```python
from build123d import *

# Parameters (mm, degrees)
BOSS_EXTRUDE1_DEPTH            = 43
BOSS_EXTRUDE2_DEPTH            = 33
SKETCH6_R                      = 11
CUT_EXTRUDE1_DEPTH             = 2
SKETCH7_R                      = 2.5
CUT_EXTRUDE2_DEPTH             = 4
CBORE_FOR_M3_SHCS1_D           = 3.4
CBORE_FOR_M3_SHCS1_CBORE_D     = 6.5
CBORE_FOR_M3_SHCS1_CBORE_DEPTH = 3
CBORE_FOR_M3_SHCS2_D           = 3.4
CBORE_FOR_M3_SHCS2_CBORE_D     = 6.5
CBORE_FOR_M3_SHCS2_CBORE_DEPTH = 3
CBORE_FOR_M3_SHCS3_D           = 3.4
CBORE_FOR_M3_SHCS3_CBORE_D     = 6.5
CBORE_FOR_M3_SHCS3_CBORE_DEPTH = 3


with BuildPart() as part:
    # Sketch1 → Boss-Extrude1 (new body)
    with BuildSketch(Plane.XY):
        Polygon((-51.369142857, 0), (-21.369142857, 0), (-21.369142857, 33), (21.630857143, 33), (21.630857143, 0), (51.630857143, 0), (51.630857143, 9), (25.630857143, 9), (25.630857143, 38), (-25.369142857, 38), (-25.369142857, 9), (-51.369142857, 9), align=None)
    extrude(amount=BOSS_EXTRUDE1_DEPTH)

    # Sketch5 → Boss-Extrude2 (add)
    with BuildSketch(Plane.XZ.offset(-33)):
        Polygon((-21.369142857, 43), (-18.369142857, 43), (-21.369142857, 40), align=None)
        Polygon((21.630857143, 40), (21.630857143, 43), (18.630857143, 43), align=None)
        Polygon((18.630857143, 0), (21.630857143, 0), (21.630857143, 3), align=None)
        Polygon((-18.369142857, 0), (-21.369142857, 0), (-21.369142857, 3), align=None)
    extrude(amount=BOSS_EXTRUDE2_DEPTH)

    # Sketch6 → Cut-Extrude1 (cut)
    with BuildSketch(Plane.XZ.offset(-33)):
        with Locations((0, 21.5)):
            Circle(SKETCH6_R)
    extrude(amount=-CUT_EXTRUDE1_DEPTH, mode=Mode.SUBTRACT)

    # Sketch7 → Cut-Extrude2 (cut, through all)
    with BuildSketch(Plane.XZ.offset(-35)):
        with Locations((0, 21.5)):
            Circle(SKETCH7_R)
    extrude(amount=-CUT_EXTRUDE2_DEPTH, mode=Mode.SUBTRACT)

    # CBORE for M3 SHCS1 (through all)
    with Locations(Plane(origin=(0, 38, 0), x_dir=(1, 0, 0), z_dir=(0, 1, 0))):
        with Locations((-15.369142857, -6), (-15.369142857, -37), (15.630857143, -37), (15.630857143, -6)):
            CounterBoreHole(CBORE_FOR_M3_SHCS1_D / 2, CBORE_FOR_M3_SHCS1_CBORE_D / 2, CBORE_FOR_M3_SHCS1_CBORE_DEPTH)

    # CBORE for M3 SHCS2 (through all)
    with Locations(Plane(origin=(0, 9, 0), x_dir=(1, 0, 0), z_dir=(0, 1, 0))):
        with Locations((-38.369142857, -9), (-38.369142857, -34)):
            CounterBoreHole(CBORE_FOR_M3_SHCS2_D / 2, CBORE_FOR_M3_SHCS2_CBORE_D / 2, CBORE_FOR_M3_SHCS2_CBORE_DEPTH)

    # CBORE for M3 SHCS3 (through all)
    with Locations(Plane(origin=(0, 9, 0), x_dir=(1, 0, 0), z_dir=(0, 1, 0))):
        with Locations((38.630857143, -34), (38.630857143, -9)):
            CounterBoreHole(CBORE_FOR_M3_SHCS3_D / 2, CBORE_FOR_M3_SHCS3_CBORE_D / 2, CBORE_FOR_M3_SHCS3_CBORE_DEPTH)


solid = part.part
```
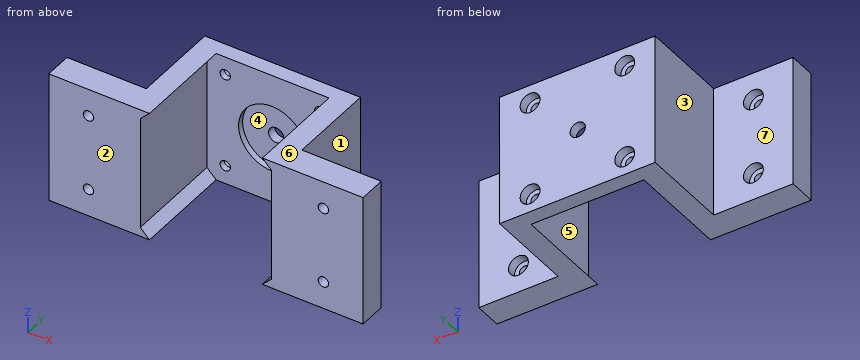
The listing builds one solid part. Answer for the finished solid, in the listing's coordinates (mm). Face numbers are marked on the shaded views. A direction names the side the tool comes from. Round coordinates to 2 decimals unless told otherwise and drop trailing zeros. Loops run counter-clockwise (first coordinate to the right, second up) from the corner with the lowest first, then second, coordinate; pieces in that order, holes last. Notation, with made-up numbers: (20.5, 53) - (74.5, 53) arc R17 cw to (74.5, 65) - close; hole circle Ø2 at (63.25, -3.5). An arc over 180 degrees is marked (long way). Return JSON: item names as keys, results as strings. Group by question number.
1. Consider probe 1 along X at (y, z) = (3, 9); probe 2 along X at (y, z) = (34.55, 6); probe 3 along X at (y, z) = (7, 34). Determine where each line is inside the solid, lowest interval first.
2. Each of these flat-tipped pins is pushed along its axis until it touches: P1, Ø8.5, axis at y = 27.5, z = 30.5, coming from the -X side; P2, Ø14.5, axis at y = 18.5, z = 22, coming from the +X side; P3, Ø17.5, axis at x = 3.5, z = 17.5, coming from the -Y side; P4, Ø5.5, axis at x = 38.63, z = 34, coming from the -Y side. Where does it stop, or does it pass through?
3. Which of the six approach directions +Z, -Z, +X, -X, +Y, -Y give full straight-line access (tool end or side, diameter ignored) to the marked faces 1, 2, 3 and 4?
4. The part is cut by section C-C on x = 0. Determine the outline of the cut face in (y, z), then the cut area to 3 significant figures.
5. The mould has two halves that part along Z. Classify the marked faces 5, 6 and 7: pulls with the +Z half, pulls with the -Z half, needs draft (parallel to the pull), parting line crosses it, or undercut.
6. The part is cut by section B-B on z = 21.5. Determine the outline of the cut face in (x, y).
7. The part is cut by section A-A on y = 18.5. Determine the outline of the cut face in (x, z).
8. The part is cut by section D-D on x = 15. Determine the outline of the cut face in (y, z), then the cut area to 3 significant figures.
Resolved:
{
 "1": {"probe 1": "x = -51.37 to -40.07, -36.67 to -21.37, 21.63 to 36.93, 40.33 to 51.63", "probe 2": "x = -25.37 to -17.07, -13.67 to 13.93, 17.33 to 25.63", "probe 3": "x = -51.37 to -41.62, -35.12 to -21.37, 21.63 to 35.38, 41.88 to 51.63"},
 "2": {"P1": "stops at x = -25.37", "P2": "stops at x = 25.63", "P3": "stops at y = 33", "P4": "stops at y = 0"},
 "3": {"face 1": "+Z, -Z, +X, +Y", "face 2": "+Z, -Z, +X, -X, -Y", "face 3": "+Z, -Z, -X, +Y", "face 4": "-Y"},
 "4": {"outline": "(33, 0) - (38, 0) - (38, 19) - (35, 19) - (35, 10.5) - (33, 10.5) - close; (33, 32.5) - (35, 32.5) - (35, 24) - (38, 24) - (38, 43) - (33, 43) - close", "area": "156 mm²"},
 "5": {"face 5": "undercut", "face 6": "pulls with the +Z half", "face 7": "needs draft"},
 "6": {"outline": "(-51.37, 0) - (-21.37, 0) - (-21.37, 33) - (-11, 33) - (-11, 35) - (-2.5, 35) - (-2.5, 38) - (-25.37, 38) - (-25.37, 9) - (-51.37, 9) - close; (2.5, 35) - (11, 35) - (11, 33) - (21.63, 33) - (21.63, 0) - (51.63, 0) - (51.63, 9) - (25.63, 9) - (25.63, 38) - (2.5, 38) - close"},
 "7": {"outline": "(-25.37, 0) - (-18.37, 0) - (-21.37, 3) - (-21.37, 40) - (-18.37, 43) - (-25.37, 43) - close; (18.63, 0) - (25.63, 0) - (25.63, 43) - (18.63, 43) - (21.63, 40) - (21.63, 3) - close"},
 "8": {"outline": "(33, 0) - (38, 0) - (38, 2.81) - (35, 2.81) - (35, 4.42) - (33, 4.42) - close; (33, 7.58) - (35, 7.58) - (35, 9.19) - (38, 9.19) - (38, 33.81) - (35, 33.81) - (35, 35.42) - (33, 35.42) - close; (33, 38.58) - (35, 38.58) - (35, 40.19) - (38, 40.19) - (38, 43) - (33, 43) - close", "area": "164 mm²"}
}
